Can you work these out from the model? Positions are in its coordinate system, mm. A direction names the side the tool comes from. Round coordinates to 2 decimals unless told otherwise and drop trailing zeros. Write each loop counter-clockwise with the first axis right and the second up, starting at its lowest first coordinate (ties: lowest second). Pieces come first, ordered by that corner, then holes. Notation, with made-up numbers: M 54.25,28.25 L 64.25,28.25 A31 ccw 64.25,53.25 Z; hole C -23.75,-34 d7. An arc over 180 degrees is marked long. Answer in a Markdown table with one row per item. Add a question column.
(1) Suppose I cut it at A-A, the plane z = 164. Write out the boundary of the cut face in (x, y), then the cut area to 3 significant figures.
(2) I'm going to push flat-ended pins straight in: pin 1 (4 mm diameter, centred on y = -2.5, z = 11, fed in from +X); pin 2 (2 mm diameter, centred on y = 2, z = 111.5, fed in from +X). Where does each tip first touch, or does it pass through?
(3) Suppose I cut it at B-B, the plane x = -1.5. Write out the boundary of the cut face in (y, z), then the cut area to 3 significant figures.
(4) If we mould it in two halves opening along Y, with no side actions, what happens to faces 1 (the face through (0, -4, 164)), 2 (the face through (-3, 3, 160)), 3 (the face through (-0.06, -0.62, 162.03)), 4 (the face through (0, 4, -4))? For each: released by +Y, released by -Y, zero draft, split by the parting line, or undercut.
(5) For faces 5 (the face through (3, -3, 0)), 6 (the face through (-3, 3, 0)), 7 (the face through (-3, -3, 0)), 8 (the face through (-0.867, 3.905, 78.88)), which set-ups out of +Z, -Z, +X, -X, +Y, -Y let a thin tool reach every point of the face, with its end or its side?
(6) If I drill on probe 1 along Z at (x, y) = (-2.75, -0.5); probe 2 along Z at (x, y) = (0.75, -0.25); probe 3 along Y at (x, z) = (-0.5, 164), over which ranges is the centre line in solid material (lowest first)?
(7) Suppose I cut it at C-C, the plane z = 54.5. Write out the boundary of the cut face in (x, y), then the cut area to 3 significant figures.
Autodesk Inventor part; units mm, degrees
ref_plane "YZ Plane" through (0, 0, 0) normal (1, 0, 0) x (0, 1, 0)
ref_plane "XZ Plane" through (0, 0, 0) normal (0, 1, 0) x (-1, 0, 0)
ref_plane "XY Plane" through (0, 0, 0) normal (0, 0, 1) x (1, 0, 0)
sketch "Szkic1" plane through (0, 0, 0) normal (0, 0, 1) x (1, 0, 0)
  circle A0 centre (0, 0) radius 4
  dimension "d0" = 8
extrude "Wyciągnięcie proste1" add sketch "Szkic1" along normal blind 160
sketch "Szkic2" plane through (0, 0, 160) normal (0, 0, 1) x (1, 0, 0)
  line L0 (4, -4) -> (-4, -4)
  line L1 (-4, -4) -> (-4, 4)
  line L2 (-4, 4) -> (4, 4)
  line L3 (4, 4) -> (4, -4)
  line L4 (4, -4) -> (-4, 4) construction
  line L5 (-4, -4) -> (4, 4) construction
  point P0 (0, 0)
  dimension "d3" = 8
  dimension "d4" = 8
extrude "Wyciągnięcie proste2" add sketch "Szkic2" along normal blind 8
sketch "Szkic3" plane through (0, 0, 0) normal (0, 0, -1) x (-1, 0, 0)
  line L0 (4, -4) -> (-4, -4)
  line L1 (4, 4) -> (-4, 4)
  line L2 (-4, 4) -> (-4, -4)
  line L3 (-4, -4) -> (4, -4)
  line L4 (4, -4) -> (4, 4)
  line L5 (4, 4) -> (-4, -4) construction
  line L6 (-4, 4) -> (4, -4) construction
  point P0 (0, 0)
extrude "Wyciągnięcie proste3" add sketch "Szkic3" along normal blind 8
sketch "Szkic4" plane through (4, 0, 0) normal (1, 0, 0) x (0, 0, -1)
  line L0 (0, -4) -> (8, -4) construction
  line L1 (8, -4) -> (0, 3.9612) construction
  line L2 (0, 0) -> (0, -4) construction
  line L3 (8, -4) -> (8, 4) construction
  line L4 (0, -4) -> (8, 4) construction
  line L5 (-160, 0) -> (-160, -4) construction
  line L6 (-168, 4) -> (-168, -4) construction
  line L7 (-160, -4) -> (-168, 4) construction
  line L8 (-168, 4) -> (-168, -4) construction
  line L9 (-168, -4) -> (-160, 4) construction
sketch "Szkic5" plane through (4, 0, 0) normal (1, 0, 0) x (0, 0, -1)
  point P0 (0, 0)
  point P1 (3.9975, -0.0288)
hole "Otwór1" at (4, -0.0288, -3.9975) direction (-1, 0, 0) diameter 4.134 end through all
sketch "Szkic6" plane through (4, -4, 160) normal (1, 0, 0) x (0, 0, -1)
  point P0 (160, 4)
  point P1 (-4, 3.9995)
hole "Otwór2" at (4, -0.0005, 164) direction (-1, 0, 0) diameter 4.134 end through all
properties part number "wal_sr_tyl"
Calculated:
| question | item | result |
|---|---|---|
| 1 | outline | M -4,-4 L 4,-4 L 4,-2.07 L -4,-2.07 Z; M -4,2.07 L 4,2.07 L 4,4 L -4,4 Z |
| 1 | area | 30.9 mm² |
| 2 | pin 1 | x = 3.97 |
| 2 | pin 2 | x = 3.87 |
| 3 | outline | M -4,-8 L 4,-8 L 4,0 L 3.71,0 L 3.71,160 L 4,160 L 4,168 L -4,168 L -4,160 L -3.71,160 L -3.71,0 L -4,0 Z; hole C -0.03,-4 d4.13; hole C 0,164 d4.13 |
| 3 | area | 1,290 mm² |
| 4 | face 1 | released by -Y |
| 4 | face 2 | zero draft |
| 4 | face 3 | undercut |
| 4 | face 4 | released by +Y |
| 5 | face 5 | +X, -Y |
| 5 | face 6 | -X, +Y |
| 5 | face 7 | -X, -Y |
| 5 | face 8 | none |
| 6 | probe 1 | -8 to -6.01, -1.98 to 161.99, 166.01 to 168 |
| 6 | probe 2 | -8 to -6.05, -1.94 to 161.95, 166.05 to 168 |
| 6 | probe 3 | -4 to -2.07, 2.07 to 4 |
| 7 | outline | C 0,0 d8 |
| 7 | area | 50.3 mm² |
